Design review of the part built by this model. Coordinates are the model's own, in mm. A direction names the side the tool comes from. Coordinates: 2 decimals unless noted, no trailing zeros. Loops run counter-clockwise (first coordinate to the right, second up) from the corner with the lowest first, then second, coordinate; pieces in that order, holes last.
Q1. For P1, Ø1, axis at x = -68, z = -25, coming from the -Y side (3 decimals); P2, Ø3, axis at y = -16, z = -20.5, coming from the +X side, all flat-tipped, find the tip position at first contact; note any pin that passes through.
Q2. Add section D-D on z = 29.5. Give the boundary of the cut face in (x, y) (3 decimals), and give its area (3 significant figures).
Q3. Draft analysis for pull direction Z (two halves, no side actions). For faces 3 (the face through (32.409, -8, -1)), 4 (the face through (29.234, -5, 0)), 5 (the face through (-35, -8, -50.612)), state which applies: released by +Z, released by -Z, zero draft, split by the parting line, or undercut.
Q4. Wall thickness on probe 1 along X at (y, z) = (-5.5, 36); probe 2 along Z at (x, y) = (-40, -4.75); probe 3 along Y at (x, z) = (-45.5, -40.5) (3 decimals): over which ranges is each line inside the solid? List them lowest first.
Q5. Add section A-A on y = -10.5. Give the boundary of the cut face in (x, z) (3 decimals), and give its area (3 significant figures).
Q6. Add section C-C on x = -32. Give the boundary of the cut face in (y, z) (3 decimals).
Q7. Add section B-B on z = 0. Give the boundary of the cut face in (x, y) (3 decimals), and give its area (3 significant figures).
Q8. Machinability: for faces 1 (the face through (-12, -6.35, 2)), 2 (the face through (-35, 0, 1)), which of the approach directions +Z, -Z, +X, -X, +Y, -Y give a long, thin tool a straight path to every point of the face, cutting with its end or side? Answer none if there is none.
```python
from build123d import *

# Parameters (mm, degrees)
F0_W         = 133.35
F0_H         = 101.6
F1_DEPTH     = 19.05
F2_T         = -3.175
F3_R         = 6.35
F4_DEPTH     = 3.175
F5_R         = 3.175
F6_DEPTH     = 12.7
F7_R         = 3.175
F8_DEPTH     = 12.7
F9_T1_DEPTH  = 95.25
F9_T3_DEPTH  = 127
F9_T9_DEPTH  = 158.75
F9_T15_DEPTH = 127
F9_T24_DEPTH = 158.75
F9_T30_DEPTH = 127
F9_T39_DEPTH = 127
F9_T45_DEPTH = 158.75
F9_T54_DEPTH = 158.75
F9_T60_DEPTH = 127
F10_SIZE     = 1.6002


# Not quite as in the source:
# - a fillet or chamfer that OpenCascade refuses, or shapes differently, is made with other operations: its cross-section is extruded or revolved along the edge and cut away or added


with BuildPart() as f1:
    # F0 (on Front) → F1 (new body)
    with BuildSketch(Plane.XZ):
        with Locations((-34.2663429767, 0.1884810627)):
            Rectangle(F0_W, F0_H)
    extrude(amount=F1_DEPTH)

    # F2
    f2_openings = [f1.faces().sort_by_distance(p)[0] for p in [
        (-34.266343, -19.05, 0.188481),
    ]]
    offset(amount=F2_T, openings=f2_openings)

    # F3 (on face) → F4 (join)
    with BuildSketch(Plane.XZ.offset(3.175)):
        with Locations((-66.0163429767, 0)):
            Circle(F3_R)
        with Locations((-8.8663429767, 0)):
            Circle(F3_R)
    extrude(amount=F4_DEPTH)

    # F5 (on face) → F6 (join)
    with BuildSketch(Plane.XZ.offset(6.35)):
        with Locations((-66.0163429767, 0)):
            Circle(F5_R)
    extrude(amount=F6_DEPTH)

    # F7 (on face) → F8 (join)
    with BuildSketch(Plane.XZ.offset(6.35)):
        with Locations((-8.8663429767, 0)):
            Circle(F7_R)
    extrude(amount=F8_DEPTH)

    # F9: fillet of radius 12.7 on 4 edges, made by hand

    # F9_s2 → F9_t1 (cut)
    with BuildSketch(Plane.XY.offset(-47.4365189373)):
        with BuildLine():
            ThreePointArc((-110.4663429767, -19.05), (-101.4860868556, -15.3302561211), (-97.7663429767, -6.35))
            Line((-97.7663429767, -6.35), (-97.7663429767, -19.05))
            Line((-97.7663429767, -19.05), (-110.4663429767, -19.05))
        make_face()
        with BuildLine():
            ThreePointArc((41.9336570233, -19.05), (32.9534009023, -15.3302561211), (29.2336570233, -6.35))
            Line((29.2336570233, -6.35), (29.2336570233, -19.05))
            Line((29.2336570233, -19.05), (41.9336570233, -19.05))
        make_face()
    extrude(amount=F9_T1_DEPTH, mode=Mode.SUBTRACT)

    # F9_s4 → F9_t3 (cut)
    with BuildSketch(Plane.YZ.offset(-97.7663429767)):
        with BuildLine():
            ThreePointArc((-19.05, -60.1365189373), (-15.3302561211, -51.1562628163), (-6.35, -47.4365189373))
            Line((-6.35, -47.4365189373), (-19.05, -47.4365189373))
            Line((-19.05, -47.4365189373), (-19.05, -60.1365189373))
        make_face()
        with BuildLine():
            ThreePointArc((-19.05, 60.5134810627), (-15.3302561211, 51.5332249416), (-6.35, 47.8134810627))
            Line((-6.35, 47.8134810627), (-19.05, 47.8134810627))
            Line((-19.05, 47.8134810627), (-19.05, 60.5134810627))
        make_face()
    extrude(amount=F9_T3_DEPTH, mode=Mode.SUBTRACT)


with BuildPart() as f9_tool7:
    # F9_s8 → F9_t9 (new body)
    with BuildSketch(Plane.YZ.offset(29.2336570233)):
        with BuildLine():
            ThreePointArc((-19.05, 60.5134810627), (-15.3302561211, 51.5332249416), (-6.35, 47.8134810627))
            Line((-6.35, 47.8134810627), (-19.05, 47.8134810627))
            Line((-19.05, 47.8134810627), (-19.05, 60.5134810627))
        make_face()
    extrude(amount=-F9_T9_DEPTH)

    split(bisect_by=Plane.XY.offset(50.9884810627), keep=Keep.BOTTOM)

    split(bisect_by=Plane.YZ.offset(-100.9413429767), keep=Keep.TOP)

    split(bisect_by=Plane.YZ.offset(-97.7663429767), keep=Keep.BOTTOM)


with BuildPart() as f9_tool13:
    # F9_s14 → F9_t15 (new body)
    with BuildSketch(Plane.XY.offset(79.5634810627)):
        with BuildLine():
            ThreePointArc((-110.4663429767, -19.05), (-101.4860868556, -15.3302561211), (-97.7663429767, -6.35))
            Line((-97.7663429767, -6.35), (-97.7663429767, -19.05))
            Line((-97.7663429767, -19.05), (-110.4663429767, -19.05))
        make_face()
    extrude(amount=-F9_T15_DEPTH)

    split(bisect_by=Plane.XY.offset(50.9884810627), keep=Keep.BOTTOM)

    split(bisect_by=Plane.YZ.offset(-100.9413429767), keep=Keep.TOP)

    split(bisect_by=Plane.XY.offset(47.8134810627), keep=Keep.TOP)


with BuildPart() as f9_tool7_1:
    add(f9_tool7.part)

    # F9_t19: intersect F9_tool13
    add(f9_tool13.part, mode=Mode.INTERSECT)


with BuildPart() as f1_1:
    add(f1.part)

    # F9_t5: cut F9_tool7
    add(f9_tool7_1.part, mode=Mode.SUBTRACT)


with BuildPart() as f9_tool22:
    # F9_s23 → F9_t24 (new body)
    with BuildSketch(Plane.YZ.offset(-129.5163429767)):
        with BuildLine():
            ThreePointArc((-19.05, -60.1365189373), (-15.3302561211, -51.1562628163), (-6.35, -47.4365189373))
            Line((-6.35, -47.4365189373), (-19.05, -47.4365189373))
            Line((-19.05, -47.4365189373), (-19.05, -60.1365189373))
        make_face()
    extrude(amount=F9_T24_DEPTH)

    split(bisect_by=Plane.YZ.offset(-100.9413429767), keep=Keep.TOP)

    split(bisect_by=Plane.XY.offset(-50.6115189373), keep=Keep.TOP)

    split(bisect_by=Plane.YZ.offset(-97.7663429767), keep=Keep.BOTTOM)


with BuildPart() as f9_tool28:
    # F9_s29 → F9_t30 (new body)
    with BuildSketch(Plane.XY.offset(47.8134810627)):
        with BuildLine():
            ThreePointArc((-110.4663429767, -19.05), (-101.4860868556, -15.3302561211), (-97.7663429767, -6.35))
            Line((-97.7663429767, -6.35), (-97.7663429767, -19.05))
            Line((-97.7663429767, -19.05), (-110.4663429767, -19.05))
        make_face()
    extrude(amount=-F9_T30_DEPTH)

    split(bisect_by=Plane.YZ.offset(-100.9413429767), keep=Keep.TOP)

    split(bisect_by=Plane.XY.offset(-50.6115189373), keep=Keep.TOP)

    split(bisect_by=Plane.XY.offset(-47.4365189373), keep=Keep.BOTTOM)


with BuildPart() as f9_tool22_1:
    add(f9_tool22.part)

    # F9_t34: intersect F9_tool28
    add(f9_tool28.part, mode=Mode.INTERSECT)


with BuildPart() as f1_2:
    add(f1_1.part)

    # F9_t20: cut F9_tool22
    add(f9_tool22_1.part, mode=Mode.SUBTRACT)


with BuildPart() as f9_tool37:
    # F9_s38 → F9_t39 (new body)
    with BuildSketch(Plane.XY.offset(-79.1865189373)):
        with BuildLine():
            ThreePointArc((41.9336570233, -19.05), (32.9534009023, -15.3302561211), (29.2336570233, -6.35))
            Line((29.2336570233, -6.35), (29.2336570233, -19.05))
            Line((29.2336570233, -19.05), (41.9336570233, -19.05))
        make_face()
    extrude(amount=F9_T39_DEPTH)

    split(bisect_by=Plane.YZ.offset(32.4086570233), keep=Keep.BOTTOM)

    split(bisect_by=Plane.XY.offset(-50.6115189373), keep=Keep.TOP)

    split(bisect_by=Plane.XY.offset(-47.4365189373), keep=Keep.BOTTOM)


with BuildPart() as f9_tool43:
    # F9_s44 → F9_t45 (new body)
    with BuildSketch(Plane.YZ.offset(-97.7663429767)):
        with BuildLine():
            ThreePointArc((-19.05, -60.1365189373), (-15.3302561211, -51.1562628163), (-6.35, -47.4365189373))
            Line((-6.35, -47.4365189373), (-19.05, -47.4365189373))
            Line((-19.05, -47.4365189373), (-19.05, -60.1365189373))
        make_face()
    extrude(amount=F9_T45_DEPTH)

    split(bisect_by=Plane.YZ.offset(32.4086570233), keep=Keep.BOTTOM)

    split(bisect_by=Plane.XY.offset(-50.6115189373), keep=Keep.TOP)

    split(bisect_by=Plane.YZ.offset(29.2336570233), keep=Keep.TOP)


with BuildPart() as f9_tool37_1:
    add(f9_tool37.part)

    # F9_t49: intersect F9_tool43
    add(f9_tool43.part, mode=Mode.INTERSECT)


with BuildPart() as f1_3:
    add(f1_2.part)

    # F9_t35: cut F9_tool37
    add(f9_tool37_1.part, mode=Mode.SUBTRACT)


with BuildPart() as f9_tool52:
    # F9_s53 → F9_t54 (new body)
    with BuildSketch(Plane.YZ.offset(60.9836570233)):
        with BuildLine():
            ThreePointArc((-19.05, 60.5134810627), (-15.3302561211, 51.5332249416), (-6.35, 47.8134810627))
            Line((-6.35, 47.8134810627), (-19.05, 47.8134810627))
            Line((-19.05, 47.8134810627), (-19.05, 60.5134810627))
        make_face()
    extrude(amount=-F9_T54_DEPTH)

    split(bisect_by=Plane.XY.offset(50.9884810627), keep=Keep.BOTTOM)

    split(bisect_by=Plane.YZ.offset(32.4086570233), keep=Keep.BOTTOM)

    split(bisect_by=Plane.YZ.offset(29.2336570233), keep=Keep.TOP)


with BuildPart() as f9_tool58:
    # F9_s59 → F9_t60 (new body)
    with BuildSketch(Plane.XY.offset(-47.4365189373)):
        with BuildLine():
            ThreePointArc((41.9336570233, -19.05), (32.9534009023, -15.3302561211), (29.2336570233, -6.35))
            Line((29.2336570233, -6.35), (29.2336570233, -19.05))
            Line((29.2336570233, -19.05), (41.9336570233, -19.05))
        make_face()
    extrude(amount=F9_T60_DEPTH)

    split(bisect_by=Plane.XY.offset(50.9884810627), keep=Keep.BOTTOM)

    split(bisect_by=Plane.YZ.offset(32.4086570233), keep=Keep.BOTTOM)

    split(bisect_by=Plane.XY.offset(47.8134810627), keep=Keep.TOP)


with BuildPart() as f9_tool52_1:
    add(f9_tool52.part)

    # F9_t64: intersect F9_tool58
    add(f9_tool58.part, mode=Mode.INTERSECT)


with BuildPart() as f1_4:
    add(f1_3.part)

    # F9_t50: cut F9_tool52
    add(f9_tool52_1.part, mode=Mode.SUBTRACT)

    # F10
    f10_edges = [f1_4.edges().sort_by_distance(p)[0] for p in [
        (-34.266343, 0, 50.988481),
        (-100.941343, 0, 0.188481),
        (-34.266343, 0, -50.611519),
        (32.408657, 0, 0.188481),
    ]]
    chamfer(f10_edges, length=F10_SIZE)


solid = f1_4.part
```
Entries:
1. P1: stops at y = -3.175
1. P2: stops at x = 32.41
2. outline: (-100.941, -14.75) arc R12.7 ccw to (-97.766, -6.35) - (-97.766, -3.175) - (29.234, -3.175) - (29.234, -6.35) arc R12.7 ccw to (32.409, -14.75) - (32.409, -1.6) - (30.808, 0) - (-99.341, 0) - (-100.941, -1.6) - close
2. area: 478 mm2
3. face 3: zero draft
3. face 4: undercut
3. face 5: released by -Z
4. probe 1: x = -100.94 to -97.77, 29.23 to 32.41
4. probe 2: z = -50.61 to -47.44, 47.81 to 50.99
4. probe 3: y = -3.175 to 0
5. outline: (-100.941, -50.612) - (32.409, -50.612) - (32.409, 50.988) - (-100.941, 50.988) - close; circle Ø6.35 at (-66.016, 0); circle Ø6.35 at (-8.866, 0); hole (-98.464, -48.134) - (29.931, -48.134) - (29.931, 48.511) - (-98.464, 48.511) - close
5. area: 1,200 mm2
6. outline: (-14.75, -50.612) - (-1.6, -50.612) - (0, -49.011) - (0, 49.388) - (-1.6, 50.988) - (-14.75, 50.988) arc R12.7 ccw to (-6.35, 47.813) - (-3.175, 47.813) - (-3.175, -47.437) - (-6.35, -47.437) arc R12.7 ccw to start
7. outline: (-100.941, -14.75) arc R12.7 ccw to (-97.766, -6.35) - (-97.766, -3.175) - (-72.366, -3.175) - (-72.366, -6.35) - (-69.191, -6.35) - (-69.191, -19.05) - (-62.841, -19.05) - (-62.841, -6.35) - (-59.666, -6.35) - (-59.666, -3.175) - (-15.216, -3.175) - (-15.216, -6.35) - (-12.041, -6.35) - (-12.041, -19.05) - (-5.691, -19.05) - (-5.691, -6.35) - (-2.516, -6.35) - (-2.516, -3.175) - (29.234, -3.175) - (29.234, -6.35) arc R12.7 ccw to (32.409, -14.75) - (32.409, -1.6) - (30.808, 0) - (-99.341, 0) - (-100.941, -1.6) - close
7. area: 719 mm2
8. face 1: -Y
8. face 2: +Z, -Z, +X, -X, +Y
